```python
from build123d import *

# Parameters (mm, degrees)
F0_W     = 38.1
F0_H     = 38.1
F2_DEPTH = 25.4
F3_D     = 3.6322
F4_D     = 3.6576
F5_D     = 3.6068
F6_D     = 3.683


with BuildPart() as f2:
    # F0 (on Front) → F2 (new body)
    with BuildSketch(Plane.XZ):
        with Locations((19.05, -19.05)):
            Rectangle(F0_W, F0_H)
    extrude(amount=F2_DEPTH)

    # F3 (through all)
    with Locations(Plane(origin=(0, 0, 0), x_dir=(1, 0, 0), z_dir=(0, 1, 0))):
        with Locations((9.525, 9.525)):
            Hole(F3_D / 2)

    # F4 (through all)
    with Locations(Plane(origin=(0, 0, 0), x_dir=(1, 0, 0), z_dir=(0, 1, 0))):
        with Locations((28.575, 9.525)):
            Hole(F4_D / 2)

    # F5 (through all)
    with Locations(Plane(origin=(0, 0, 0), x_dir=(1, 0, 0), z_dir=(0, 1, 0))):
        with Locations((9.525, 28.575)):
            Hole(F5_D / 2)

    # F6 (through all)
    with Locations(Plane(origin=(0, 0, 0), x_dir=(1, 0, 0), z_dir=(0, 1, 0))):
        with Locations((28.575, 28.575)):
            Hole(F6_D / 2)


solid = f2.part
```
Geometry: final body of the model. Coordinates: model frame, mm. Round coordinates to 2 decimals unless told otherwise and drop trailing zeros. Loops run counter-clockwise (first coordinate to the right, second up) from the corner with the lowest first, then second, coordinate; pieces in that order, holes last.
Item 1: Section A-A, the plane x = 27.5. Output: boundary loops of the cut face in (y, z), plus the area to 3 significant figures.
Checked values:
outline: (-25.4, -38.1) - (0, -38.1) - (0, -30.07) - (-25.4, -30.07) - close; (-25.4, -27.08) - (0, -27.08) - (0, -11) - (-25.4, -11) - close; (-25.4, -8.05) - (0, -8.05) - (0, 0) - (-25.4, 0) - close
area: 817 mm2
Item 2: Contact query for a flat-ended pin moving along its axis: P1, Ø5, axis at x = 28.575, z = -28.575, coming from the +Y side. Output: stop coordinate, or through.
Checked values:
P1: stops at y = 0
Item 3: Section B-B, the plane y = -16. Output: boundary loops of the cut face in (x, z) (1 decimal).
Checked values:
outline: (0, -38.1) - (38.1, -38.1) - (38.1, 0) - (0, 0) - close; hole circle Ø3.6 at (9.5, -28.6); hole circle Ø3.6 at (9.5, -9.5); hole circle Ø3.7 at (28.6, -28.6); hole circle Ø3.7 at (28.6, -9.5)
Item 4: Mould query, pull axis Z, two halves, no side actions, for faces 1 (the cylindrical face through (7.847, -12.878, -8.829)), 2 (the flat face through (19, -13, -38.1)), 3 (the flat face through (19, 0, -19)). Classes: released by +Z, released by -Z, zero draft, split by the parting line, or undercut.
Checked values:
face 1: undercut
face 2: released by -Z
face 3: zero draft
Item 5: Line query: L1, parallel to Z at x = 28.5, y = -14.75; L2, parallel to Z at x = 11, y = -18.5; L3, parallel to X at y = -10.5, z = -10. Output: solid intervals per line, ascending.
Checked values:
L1: z = -38.1 to -30.41, -26.74 to -11.35, -7.7 to 0
L2: z = -38.1 to -29.61, -27.54 to -10.58, -8.47 to 0
L3: x = 0 to 7.77, 11.28 to 26.81, 30.34 to 38.1
